Check sheet for the modelled part. Datum: model origin and axes. Units: mm. Coordinates: 2 decimals unless noted, no trailing zeros. Loops run counter-clockwise (first coordinate to the right, second up) from the corner with the lowest first, then second, coordinate; pieces in that order, holes last. Notation, with made-up numbers: (10, 52) - (49, 52) arc R12 ccw to (49, 73) - close; hole circle Ø8 at (1.5, 8.5). An arc over 180 degrees is marked (long way). Use a Markdown table: item, result. Add a question column.
1) Sectioned sample at A-A, the plane x = 13.25. Enter the section's corners in (y, z), then the cut area to 3 significant figures.
2) Sectioned sample at B-B, the plane y = 103.5. Enter the section's corners in (x, z), then the cut area to 3 significant figures.
3) Thickness scan on line 1 (Y direction, x = 19.6, z = 28) (3 decimals); line 2 (Z direction, x = 0.7, y = 982) (3 decimals); line 3 (X direction, y = 535.5, z = 23.5). Record the ranges inside material, lowest first.
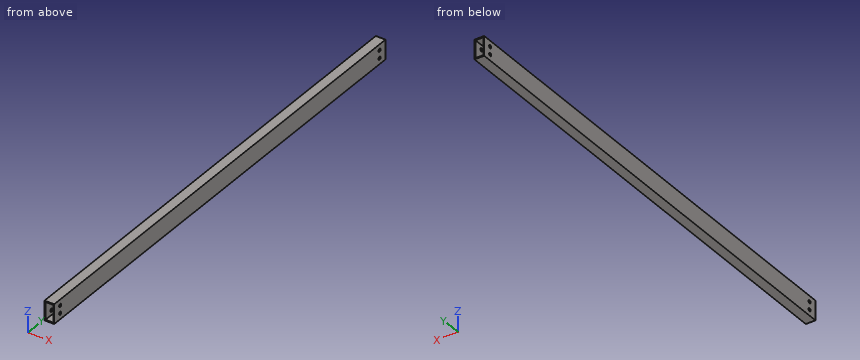
from build123d import *

# Parameters (mm, degrees)
CROQUIS1_W              = 40
CROQUIS1_H              = 1000
SALIENTE_EXTRUIR1_DEPTH = 20
CROQUIS2_W              = 16
CROQUIS2_H              = 36
CORTAR_EXTRUIR1_DEPTH   = 1000
CROQUIS3_R              = 3.175
CORTAR_EXTRUIR2_DEPTH   = 1000


with BuildPart() as part:
    # Croquis1 → Saliente-Extruir1 (new body)
    with BuildSketch(Plane(origin=(0, 0, 0), x_dir=(0, 0, -1), z_dir=(1, 0, 0))):
        with Locations((-20, 500)):
            Rectangle(CROQUIS1_W, CROQUIS1_H)
    extrude(amount=SALIENTE_EXTRUIR1_DEPTH)

    # Croquis2 → Cortar-Extruir1 (cut)
    with BuildSketch(Plane(origin=(0, 1000, 0), x_dir=(1, 0, 0), z_dir=(0, 1, 0))):
        with Locations((10, -20)):
            Rectangle(CROQUIS2_W, CROQUIS2_H)
    extrude(amount=-CORTAR_EXTRUIR1_DEPTH, mode=Mode.SUBTRACT)

    # Croquis3 → Cortar-Extruir2 (cut)
    with BuildSketch(Plane.ZY):
        with Locations((12, 982)):
            Circle(CROQUIS3_R)
        with Locations((28, 982)):
            Circle(CROQUIS3_R)
        with Locations((28, 18)):
            Circle(CROQUIS3_R)
        with Locations((12, 18)):
            Circle(CROQUIS3_R)
    extrude(amount=-CORTAR_EXTRUIR2_DEPTH, mode=Mode.SUBTRACT)


solid = part.part
Solved:
| question | item | result |
|---|---|---|
| 1 | outline | (0, 0) - (1000, 0) - (1000, 2) - (0, 2) - close; (0, 38) - (1000, 38) - (1000, 40) - (0, 40) - close |
| 1 | area | 4,000 mm2 |
| 2 | outline | (0, 0) - (20, 0) - (20, 40) - (0, 40) - close; hole (2, 2) - (18, 2) - (18, 38) - (2, 38) - close |
| 2 | area | 224 mm2 |
| 3 | line 1 | y = 0 to 14.825, 21.175 to 978.825, 985.175 to 1000 |
| 3 | line 2 | z = 0 to 8.825, 15.175 to 24.825, 31.175 to 40 |
| 3 | line 3 | x = 0 to 2, 18 to 20 |
